Work out the finished part from the listing and answer in its coordinate system (mm). Face numbers are marked on the shaded views. A direction names the side the tool comes from. Round coordinates to 2 decimals unless told otherwise and drop trailing zeros. Write each loop counter-clockwise with the first axis right and the second up, starting at its lowest first coordinate (ties: lowest second). Pieces come first, ordered by that corner, then holes.
1. Find section A-A (x = -33). Write down the section's boundary in (y, z).
2. Straight lines are drawn through the part: probe 1 along X at (y, z) = (12.8, 7); probe 2 along Z at (x, y) = (-33, 13.3); probe 3 along X at (y, z) = (13.1, 53). For each, find the intervals that lie inside material, in ascending order.
3. Find section D-D (x = 3). Write down the section's boundary in (y, z).
4. A tool of negligible diameter and unlimited length cuts with its end or side. For the marked faces 1, 2 and 3, from which of +Z, -Z, +X, -X, +Y, -Y can it reach the whole face along a straight path? Write none if from no direction.
5. Flat-ended cylindrical pins translate along their axes: pin 1 Ø6 at (x, y) = (-12, -10) entering from +Z; pin 2 Ø5.5 at (x, z) = (33, 53) entering from -Y; pin 3 Ø2 at (x, y) = (-5.66, 5.66) entering from +Z; pin 4 Ø3.5 at (x, z) = (-33, 53) entering from -Y. Find the tip coordinate at first contact, or state that the pin passes through.
6. Find section C-C (y = 0). Write down the section's boundary in (x, z) (3 decimals).
7. Determine the mould class of the marked faces 4, 5 and 6 for opening direction Y: pulls with the +Y half, pulls with the -Y half, needs draft (parallel to the pull), parting line crosses it, or undercut.
8. Find section B-B (z = 7). Write down the section's boundary in (x, y) (3 decimals).
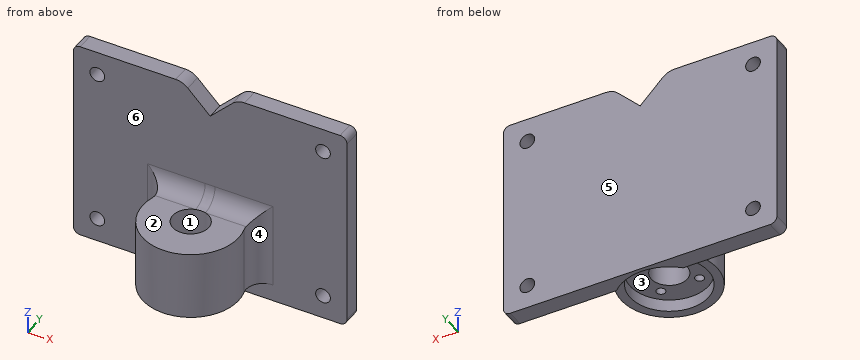
```python
from build123d import *

# Parameters (mm, degrees)
SKETCH1_R           = 5.25
BOSS_EXTRUDE1_DEPTH = 60
SKETCH2_R           = 11.425
CUT_EXTRUDE1_DEPTH  = 8.6
SKETCH3_R           = 14
CUT_EXTRUDE2_DEPTH  = 5
SKETCH4_R           = 1.3
CUT_EXTRUDE3_DEPTH  = 5
SKETCH6_R           = 2.15
CUT_EXTRUDE5_DEPTH  = 6
CUT_EXTRUDE6_DEPTH  = 35
FILLET2_R           = 5
FILLET3_R           = 2
FILLET4_R           = 5
CUT_EXTRUDE7_DEPTH  = 30.05
FILLET5_R           = 5


with BuildPart() as part:
    # Sketch1 → Boss-Extrude1 (new body)
    with BuildSketch(Plane.XY):
        with BuildLine():
            Line((-40, 15.05), (40, 15.05))
            Line((40, 15.05), (40, 10.05))
            Line((40, 10.05), (9.746666097, 10.05))
            ThreePointArc((9.746666097, 10.05), (0, -14), (-9.746666097, 10.05))
            Line((-9.746666097, 10.05), (-40, 10.05))
            Line((-40, 10.05), (-40, 15.05))
        make_face()
        Circle(SKETCH1_R, mode=Mode.SUBTRACT)
    extrude(amount=BOSS_EXTRUDE1_DEPTH)

    # Sketch2 → Cut-Extrude1 (cut)
    with BuildSketch(Plane(origin=(0, 0, 0), x_dir=(-1, 0, 0), z_dir=(0, 0, -1))):
        Circle(SKETCH2_R)
    extrude(amount=-CUT_EXTRUDE1_DEPTH, mode=Mode.SUBTRACT)

    # Sketch3 → Cut-Extrude2 (cut)
    with BuildSketch(Plane(origin=(0, 0, 0), x_dir=(-1, 0, 0), z_dir=(0, 0, -1))):
        Circle(SKETCH3_R)
    extrude(amount=-CUT_EXTRUDE2_DEPTH, mode=Mode.SUBTRACT)

    # Sketch4 → Cut-Extrude3 (cut)
    with BuildSketch(Plane(origin=(0, 0, 8.6), x_dir=(-1, 0, 0), z_dir=(0, 0, -1))):
        with Locations((5.656854249, 5.656854249)):
            Circle(SKETCH4_R)
        with Locations((5.656854249, -5.656854249)):
            Circle(SKETCH4_R)
        with Locations((-5.656854249, -5.656854249)):
            Circle(SKETCH4_R)
        with Locations((-5.656854249, 5.656854249)):
            Circle(SKETCH4_R)
    extrude(amount=-CUT_EXTRUDE3_DEPTH, mode=Mode.SUBTRACT)

    # Sketch6 → Cut-Extrude5 (cut, through all)
    with BuildSketch(Plane(origin=(0, 10.05, 0), x_dir=(-1, 0, 0), z_dir=(0, -1, 0))):
        with Locations((33, -53)):
            Circle(SKETCH6_R)
        with Locations((33, -7)):
            Circle(SKETCH6_R)
        with Locations((-33, -53)):
            Circle(SKETCH6_R)
        with Locations((-33, -7)):
            Circle(SKETCH6_R)
    extrude(amount=-CUT_EXTRUDE5_DEPTH, mode=Mode.SUBTRACT)

    # Sketch7 → Cut-Extrude6 (cut)
    with BuildSketch(Plane.XY.offset(60)):
        with BuildLine():
            Line((-9.746666097, 10.05), (9.746666097, 10.05))
            ThreePointArc((9.746666097, 10.05), (0, -14), (-9.746666097, 10.05))
        make_face()
    extrude(amount=-CUT_EXTRUDE6_DEPTH, mode=Mode.SUBTRACT)

    # Fillet2
    fillet2_edges = [part.edges().sort_by_distance(p)[0] for p in [
        (9.746666097, 10.05, 15),
        (-9.746666097, 10.05, 15),
    ]]
    fillet(fillet2_edges, radius=FILLET2_R)

    # Fillet3
    fillet3_edges = [part.edges().sort_by_distance(p)[0] for p in [
        (40, 12.55, 60),
        (-40, 12.55, 60),
        (40, 12.55, 0),
        (-40, 12.55, 0),
    ]]
    fillet(fillet3_edges, radius=FILLET3_R)

    # Fillet4
    fillet4_edges = [part.edges().sort_by_distance(p)[0] for p in [
        (0, 10.05, 25),
    ]]
    fillet(fillet4_edges, radius=FILLET4_R)

    # Sketch8 → Cut-Extrude7 (cut, through all)
    with BuildSketch(Plane(origin=(0, 15.05, 0), x_dir=(1, 0, 0), z_dir=(0, 1, 0))):
        Polygon((0, -52), (8, -60), (-8, -60), align=None)
    extrude(amount=-CUT_EXTRUDE7_DEPTH, mode=Mode.SUBTRACT)

    # Fillet5
    fillet5_edges = [part.edges().sort_by_distance(p)[0] for p in [
        (-8, 12.55, 60),
        (8, 12.55, 60),
    ]]
    fillet(fillet5_edges, radius=FILLET5_R)


solid = part.part
```
Worked answers:
1. outline: (10.05, 0) - (15.05, 0) - (15.05, 4.85) - (10.05, 4.85) - close; (10.05, 9.15) - (15.05, 9.15) - (15.05, 50.85) - (10.05, 50.85) - close; (10.05, 55.15) - (15.05, 55.15) - (15.05, 60) - (10.05, 60) - close
2. probe 1: x = -40 to -35.15, -30.85 to 30.85, 35.15 to 40
2. probe 2: z = 0 to 4.85, 9.15 to 50.85, 55.15 to 60
2. probe 3: x = -40 to -35.15, -30.85 to -1, 1 to 30.85, 35.15 to 40
3. outline: (-13.67, 5) - (-11.02, 5) - (-11.02, 8.6) - (-4.31, 8.6) - (-4.31, 25) - (-13.67, 25) - close; (4.31, 8.6) - (11.02, 8.6) - (11.02, 5) - (13.67, 5) - (13.67, 0) - (15.05, 0) - (15.05, 55) - (10.05, 55) - (10.05, 30) arc R5 cw to (5.05, 25) - (4.31, 25) - close
4. face 1: +Z, -Z
4. face 2: +Z, +X, -X, -Y
4. face 3: -Z
5. pin 1: stops at z = 25
5. pin 2: stops at y = 10.05
5. pin 3: stops at z = 25.27
5. pin 4: passes through
6. outline: (-14, 5) - (-11.425, 5) - (-11.425, 8.6) - (-5.25, 8.6) - (-5.25, 25) - (-14, 25) - close; (5.25, 8.6) - (11.425, 8.6) - (11.425, 5) - (14, 5) - (14, 25) - (5.25, 25) - close
7. face 4: undercut
7. face 5: pulls with the +Y half
7. face 6: pulls with the -Y half
8. outline: (-40, 10.05) - (-35.15, 10.05) - (-35.15, 15.05) - (-40, 15.05) - close; (-30.85, 10.05) - (-18.317, 10.05) arc R5 cw to (-13.496, 3.721) arc R14 ccw (long way) to (13.496, 3.721) arc R5 cw to (18.317, 10.05) - (30.85, 10.05) - (30.85, 15.05) - (-30.85, 15.05) - close; (35.15, 10.05) - (40, 10.05) - (40, 15.05) - (35.15, 15.05) - close; hole circle Ø22.85 at (0, 0)
